```python
from build123d import *

# Parameters (mm, degrees)
SKETCH1_W           = 874.395
SKETCH1_H           = 88.9
BOSS_EXTRUDE1_DEPTH = 25.4
CUT_EXTRUDE1_DEPTH  = 51.8


with BuildPart() as part:
    # Sketch1 → Boss-Extrude1 (new body, symmetric)
    with BuildSketch(Plane(origin=(0, 0, 0), x_dir=(1, 0, 0), z_dir=(0, 1, 0))):
        Rectangle(SKETCH1_W, SKETCH1_H)
    extrude(amount=BOSS_EXTRUDE1_DEPTH, both=True)

    # Sketch2 → Cut-Extrude1 (cut, through all)
    with BuildSketch(Plane(origin=(0, 25.4, 0), x_dir=(1, 0, 0), z_dir=(0, 1, 0))):
        Polygon((-386.3975, 44.45), (-335.5975, 5.469789011), (-284.7975, 44.45), align=None)
    extrude(amount=-CUT_EXTRUDE1_DEPTH, mode=Mode.SUBTRACT)


solid = part.part
```
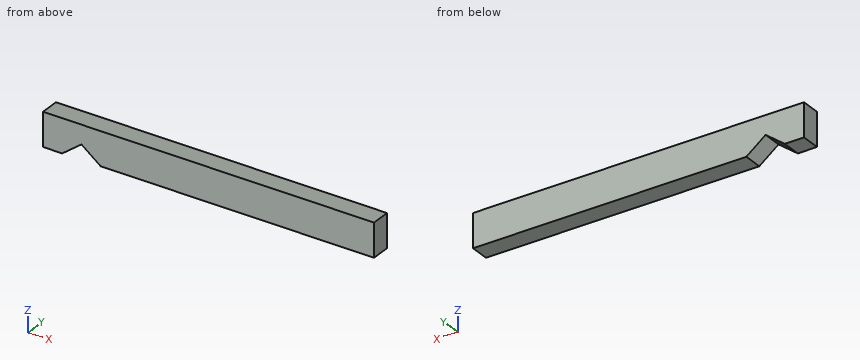
CAD build for the part. Positions are in the model's coordinates, mm. Round coordinates to 2 decimals unless told otherwise and drop trailing zeros. Order: outer loops, then holes, each group sorted by start corner. A loop starts at its lowest first (then second) coordinate and runs counter-clockwise, first axis right, second up. Notation, with made-up numbers: (-19.5, 74.25) - (-15.5, 74.25) arc R25 ccw to (-15.5, 96.25) - close; hole circle Ø11 at (-1, 62). An arc over 180 degrees is marked (long way). Answer as CSV lines item,"result". Start each with the question number.
1. Saw through at C-C, the plane x = -368.5. Write the cut outline in (y, z), and give its area (3 significant figures).
2. Saw through at B-B, the plane z = -31. Write the cut outline in (x, y), and give its area (3 significant figures).
3. Saw through at A-A, the plane y = -16.5. Write the cut outline in (x, z).
4. Drill centre lines: L1, parallel to X at y = 23.5, z = -36; L2, parallel to X at y = 10, z = -30.5; L3, parallel to Z at x = -377, y = -18. Where is each one in solid material? Low to high. Write a range as [from, to].
Model answer:
1,outline,"(-25.4, -30.72) - (25.4, -30.72) - (25.4, 44.45) - (-25.4, 44.45) - close"
1,area,"3,820 mm²"
2,outline,"(-437.2, -25.4) - (-368.87, -25.4) - (-368.87, 25.4) - (-437.2, 25.4) - close; (-302.33, -25.4) - (437.2, -25.4) - (437.2, 25.4) - (-302.33, 25.4) - close"
2,area,"41,000 mm²"
3,outline,"(-437.2, -44.45) - (-386.4, -44.45) - (-335.6, -5.47) - (-284.8, -44.45) - (437.2, -44.45) - (437.2, 44.45) - (-437.2, 44.45) - close"
4,L1,"x = [-437.2, -375.39], [-295.81, 437.2]"
4,L2,"x = [-437.2, -368.22], [-302.98, 437.2]"
4,L3,"z = [-37.24, 44.45]"
